Study the drawing (mm; zero at the part's minimum x, y, z) and answer. A direction names the side the tool comes from. Round coordinates to 2 decimals unless told otherwise and drop trailing zeros. Order: outer loops, then holes, each group sorted by start corner. A loop starts at its lowest first (then second) coordinate and runs counter-clockwise, first axis right, second up. Notation, with made-up numbers: M 9,54 L 33,54 A14 cw 33,69 Z; hole C 75.25,68 d10. An arc over 180 degrees is marked long. Put each result on its own line as item: value. Start each with the question number.
1. The part is cut by section A-A (z = 5.25). Give the vertices of the cut face in (x, y), then the cut area to 3 significant figures.
2. The mould has two halves that part along X. Classify the marked faces 4, 5, 6 and 7: +X half, -X half, draft (parallel to the pull), parting line (faces both ways), or undercut.
3. Each of these flat-tipped pins is pushed along its axis until it touches: pin 1 Ø5 at (x, y) = (35.5, 27.5) entering from -Z; pin 2 Ø3.5 at (x, z) = (15, 5.5) entering from -Y; pin 3 Ø2 at (x, z) = (1.5, 18.5) entering from -Y; pin 4 Ø1.5 at (x, y) = (27, 30) entering from +Z. Where does it stop, or does it pass through?
4. The part is cut by section B-B (y = 27). Give the vertices of the cut face in (x, z).
5. Which of the six approach directions +Z, -Z, +X, -X, +Y, -Y give full straight-line access (tool end or side, diameter ignored) to the marked faces 1, 2 and 3?
6. Consider line 1 (X direction, y = 38.7, z = 14); line 2 (X direction, y = 37, z = 13.75); line 3 (Z direction, x = 32, y = 6). Determine where each line is inside the solid, lowest interval first.
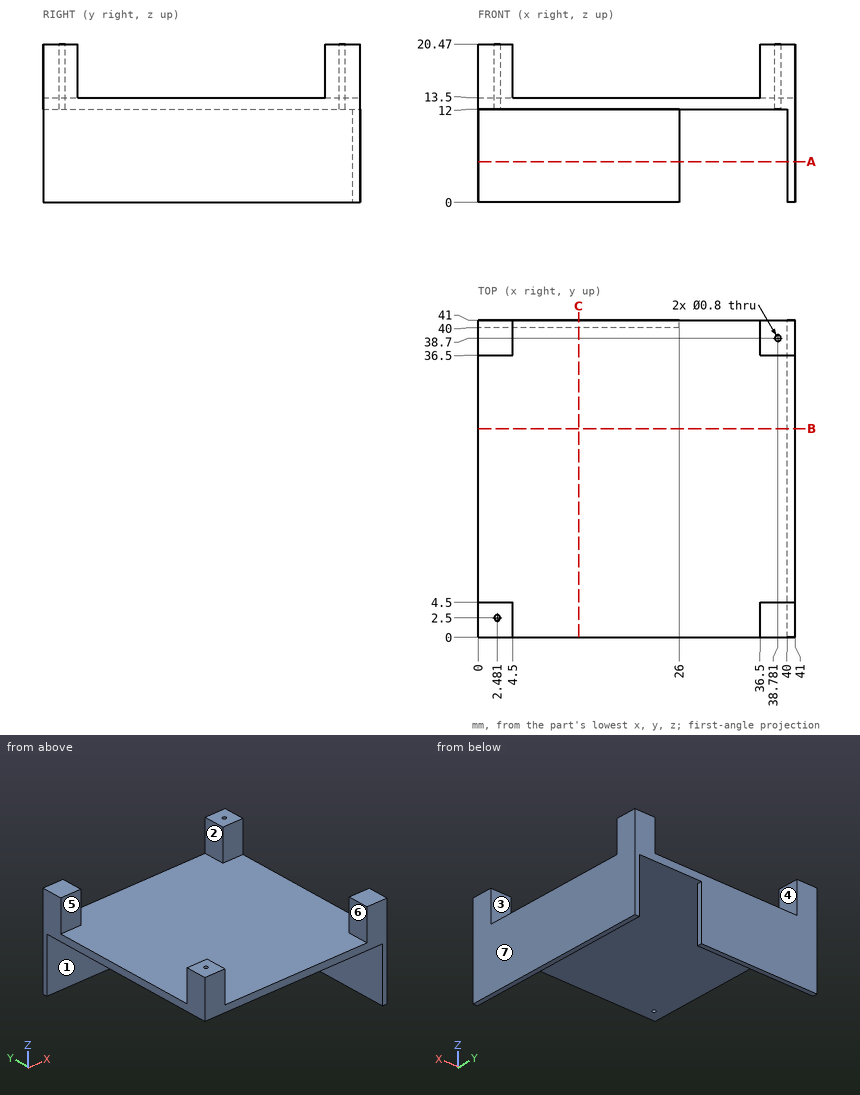
Resolved:
1. outline: M 0,40 L 26,40 L 26,41 L 0,41 Z; M 40,0 L 41,0 L 41,41 L 40,41 Z
1. area: 67.0 mm2
2. face 4: undercut
2. face 5: draft
2. face 6: undercut
2. face 7: +X half
3. pin 1: z = 12
3. pin 2: y = 40
3. pin 3: y = 0
3. pin 4: z = 13.5
4. outline: M 0,12 L 40,12 L 40,0 L 41,0 L 41,13.5 L 0,13.5 Z
5. face 1: -Z, -X, -Y
5. face 2: +Z, +Y, -Y
5. face 3: +Z, +X, -X
6. line 1: 0 to 4.5, 36.5 to 38.38, 39.18 to 41
6. line 2: 0 to 4.5, 36.5 to 41
6. line 3: 12 to 13.5
